Input: part model. Units: mm. Frame: model coordinates. Coordinates: 2 decimals unless noted, no trailing zeros. Loops run counter-clockwise (first coordinate to the right, second up) from the corner with the lowest first, then second, coordinate; pieces in that order, holes last. Notation, with made-up numbers: (19, 58) - (77, 58) arc R5 cw to (77, 64) - close; hole circle Ø4 at (19, 33). An arc over 180 degrees is marked (long way). Use one line per item in the form item = value.
from build123d import *

# Parameters (mm, degrees)
SKETCH_1_R      = 2
SKETCH_1_R_2    = 1
EXTRUDE_1_DEPTH = 25


with BuildPart() as part:
    # Эскиз1 → Бобышка-Вытянуть1 (new body)
    with BuildSketch(Plane(origin=(0, 0, 0), x_dir=(1, 0, 0), z_dir=(0, 1, 0))):
        Polygon((0, 0), (95.543981023, -9.345998627), (100.119626184, 37.430742082), (4.575645161, 46.776740709), align=None)
        with Locations(Location((4.662478276, 6.577332007, 0), (0, 0, 270))):
            Circle(SKETCH_1_R, mode=Mode.SUBTRACT)
        with Locations(Location((7.875165304, 39.420575483, 0), (0, 0, 270))):
            Circle(SKETCH_1_R, mode=Mode.SUBTRACT)
        with Locations(Location((6.26882179, 22.998953745, 0), (0, 0, 270))):
            Circle(SKETCH_1_R_2, mode=Mode.SUBTRACT)
    extrude(amount=EXTRUDE_1_DEPTH)


solid = part.part
Q1. Cut plane B-B, the plane y = 12.75. Return loops of the section in (x, z).
Check values:
outline = (0, 0) - (4.58, -46.78) - (100.12, -37.43) - (95.54, 9.35) - close; hole circle Ø4 at (4.66, -6.58); hole circle Ø2 at (6.27, -23); hole circle Ø4 at (7.88, -39.42)
Q2. Ray query, line 1 along Z through (x, y) = (7.5, 15.25); line 2 along X through (y, z) = (10.25, -8); line 3 along Z through (x, y) = (40.5, 3.25). Return the intervals inside material, ascending. Write a range as [from, to].
Check values:
line_1 = [-46.49, -41.39], [-37.46, 0.73]
line_2 = [0.78, 3.26], [6.07, 97.24]
line_3 = [-43.26, 3.96]
Q3. Cut plane C-C, the plane x = 56.5. Return loops of the section in (y, z), then the cut area to 3 significant figures.
Check values:
outline = (0, -41.7) - (25, -41.7) - (25, 5.53) - (0, 5.53) - close
area = 1,180 mm²
Q4. First-contact query: P1, Ø12, axis at y = 19, z = -26.5, coming from the +X side; P2, Ø4, axis at y = 8.5, z = -15, coming from the +X side; P3, Ø5, axis at y = 16, z = -15.5, coming from the -X side. Flat tips, straight axial feed; report the tip coordinate or a pass-through.
Check values:
P1 = 99.64
P2 = 98.12
P3 = 1.27
Q5. Cut plane A-A, the plane z = -7.5. Return loops of the section in (x, y).
Check values:
outline = (0.73, 0) - (2.89, 0) - (2.89, 25) - (0.73, 25) - close; (6.44, 0) - (97.19, 0) - (97.19, 25) - (6.44, 25) - close
Q6. Pull-direction query (X, two-part tool) for faces 1 (the flat face through (49, 25, -19)), 2 (the cylindrical face through (7.96, 12.32, -41.42)), 3 (the flat face through (47.103, 12.325, 4.608)); classes: pulls with the +X half, pulls with the -X half, needs draft (parallel to the pull), parting line crosses it, or undercut.
Check values:
face_1 = needs draft
face_2 = undercut
face_3 = pulls with the -X half
